Geometry: final body of the model. Coordinates: model frame, mm. Face numbers are marked on the shaded views. A direction names the side the tool comes from. Give positions to 0.01 mm unless a question says otherwise; leave off trailing zeros. Write each loop counter-clockwise with the first axis right and the second up, starting at its lowest first coordinate (ties: lowest second). Pieces come first, ordered by that corner, then holes.
Q1. Cut plane D-D on y = -16. Return the cut outline in (x, z).
Q2. Cut plane B-B on z = -2. Return the cut outline in (x, y).
Q3. Pin query (flat end, axial travel): pin 1 (11 mm diameter, centred on x = -47, y = 0, fed in from +Z); pin 2 (12 mm diameter, centred on x = 19.5, z = -46.5, fed in from +Y); pin 3 (14.5 mm diameter, centred on x = -48.5, y = -1, fed in from +Z); pin 4 (25 mm diameter, centred on x = 0, y = 0, fed in from +Z). Return the tip coordinate at first contact, or that it passes through.
Q4. Line query: L1, parallel to X at y = 0, z = -36; L2, parallel to Z at x = 24, y = 26.5; L3, parallel to Y at x = -47, z = -10.75. Output: solid intervals per line, ascending.
Q5. Cut plane C-C on z = -28.5. Return the cut outline in (x, y), plus the area to 3 significant figures.
Q6. Reachability of the marked faces 1, 2 and 3 from +Z, -Z, +X, -X, +Y, -Y: full face, straight path, thin tool, end or side. Return the list, or none.
Q7. Cut plane A-A on x = 0. Return the cut outline in (y, z), plus the area to 3 significant figures.
Q8. Draft query along X for the marked faces 4, 5 and 6. Return one class per face: pulls with the +X half, pulls with the -X half, needs draft (parallel to the pull), parting line crosses it, or undercut.
```python
from build123d import *

# Parameters (mm, degrees)
F0_R     = 27.5
F0_R_2   = 14
F1_DEPTH = 19
F2_DEPTH = 6
F3_R     = 27.5
F3_R_2   = 14
F4_DEPTH = 36
F5_R     = 5
F6_DEPTH = 25
F7_R     = 9
F8_DEPTH = 5


with BuildPart() as f1:
    # F0 (on Top) → F1 (new body)
    with BuildSketch(Plane.XY):
        with BuildLine():
            ThreePointArc((-33.8085106383, -9.0545352404), (-35, 0), (-33.8085106383, 9.0545352404))
            ThreePointArc((-33.8085106383, 9.0545352404), (-42.6314083028, 15.3920566067), (-53.4680851064, 14.6343389006))
            ThreePointArc((-53.4680851064, 14.6343389006), (-63, 0), (-53.4680851064, -14.6343389006))
            ThreePointArc((-53.4680851064, -14.6343389006), (-42.6314083028, -15.3920566067), (-33.8085106383, -9.0545352404))
        make_face()
        with BuildLine():
            ThreePointArc((-33.8085106383, 9.0545352404), (-26.5847239613, 22.7651587278), (-14.1489361702, 32.012616345))
            Line((-14.1489361702, 32.012616345), (-53.4680851064, 14.6343389006))
            ThreePointArc((-53.4680851064, 14.6343389006), (-42.6314083028, 15.3920566067), (-33.8085106383, 9.0545352404))
        make_face()
        with BuildLine():
            ThreePointArc((-31, 0), (-31.7182489585, 4.7400511713), (-33.8085106383, 9.0545352404))
            ThreePointArc((-33.8085106383, 9.0545352404), (-35, 0), (-33.8085106383, -9.0545352404))
            ThreePointArc((-33.8085106383, -9.0545352404), (-31.7182489585, -4.7400511713), (-31, 0))
        make_face()
        with BuildLine():
            ThreePointArc((33.8085106383, 9.0545352404), (26.5847239613, 22.7651587278), (14.1489361702, 32.012616345))
            ThreePointArc((14.1489361702, 32.012616345), (0, 35), (-14.1489361702, 32.012616345))
            ThreePointArc((-14.1489361702, 32.012616345), (-26.5847239613, 22.7651587278), (-33.8085106383, 9.0545352404))
            ThreePointArc((-33.8085106383, 9.0545352404), (-31.7182489585, 4.7400511713), (-31, 0))
            ThreePointArc((-31, 0), (-31.7182489585, -4.7400511713), (-33.8085106383, -9.0545352404))
            ThreePointArc((-33.8085106383, -9.0545352404), (-26.5847239613, -22.7651587278), (-14.1489361702, -32.012616345))
            ThreePointArc((-14.1489361702, -32.012616345), (0, -35), (14.1489361702, -32.012616345))
            ThreePointArc((14.1489361702, -32.012616345), (26.5847239613, -22.7651587278), (33.8085106383, -9.0545352404))
            ThreePointArc((33.8085106383, -9.0545352404), (31, 0), (33.8085106383, 9.0545352404))
        make_face()
        Circle(F0_R, mode=Mode.SUBTRACT)
        with BuildLine():
            ThreePointArc((-14.1489361702, -32.012616345), (-26.5847239613, -22.7651587278), (-33.8085106383, -9.0545352404))
            ThreePointArc((-33.8085106383, -9.0545352404), (-42.6314083028, -15.3920566067), (-53.4680851064, -14.6343389006))
            Line((-53.4680851064, -14.6343389006), (-14.1489361702, -32.012616345))
        make_face()
        Circle(F0_R)
        Circle(F0_R_2, mode=Mode.SUBTRACT)
        with BuildLine():
            ThreePointArc((53.4680851064, 14.6343389006), (42.6314083028, 15.3920566067), (33.8085106383, 9.0545352404))
            ThreePointArc((33.8085106383, 9.0545352404), (34.700849214, 4.5662965114), (35, 0))
            ThreePointArc((35, 0), (34.700849214, -4.5662965114), (33.8085106383, -9.0545352404))
            ThreePointArc((33.8085106383, -9.0545352404), (42.6314083028, -15.3920566067), (53.4680851064, -14.6343389006))
            ThreePointArc((53.4680851064, -14.6343389006), (60.4068893055, -8.7324291666), (63, 0))
            ThreePointArc((63, 0), (60.4068893055, 8.7324291666), (53.4680851064, 14.6343389006))
        make_face()
        with BuildLine():
            ThreePointArc((35, 0), (34.700849214, 4.5662965114), (33.8085106383, 9.0545352404))
            ThreePointArc((33.8085106383, 9.0545352404), (31, 0), (33.8085106383, -9.0545352404))
            ThreePointArc((33.8085106383, -9.0545352404), (34.700849214, -4.5662965114), (35, 0))
        make_face()
        with BuildLine():
            Line((53.4680851064, 14.6343389006), (14.1489361702, 32.012616345))
            ThreePointArc((14.1489361702, 32.012616345), (26.5847239613, 22.7651587278), (33.8085106383, 9.0545352404))
            ThreePointArc((33.8085106383, 9.0545352404), (42.6314083028, 15.3920566067), (53.4680851064, 14.6343389006))
        make_face()
        with BuildLine():
            ThreePointArc((53.4680851064, -14.6343389006), (42.6314083028, -15.3920566067), (33.8085106383, -9.0545352404))
            ThreePointArc((33.8085106383, -9.0545352404), (26.5847239613, -22.7651587278), (14.1489361702, -32.012616345))
            Line((14.1489361702, -32.012616345), (53.4680851064, -14.6343389006))
        make_face()
    extrude(amount=-F1_DEPTH)

    # F0 (on Top) → F2 (join)
    with BuildSketch(Plane.XY):
        Circle(F0_R)
        Circle(F0_R_2, mode=Mode.SUBTRACT)
    extrude(amount=F2_DEPTH)

    # F3 (on face) → F4 (join)
    with BuildSketch(Plane(origin=(0, 0, -19), x_dir=(1, 0, 0), z_dir=(0, 0, -1))):
        Circle(F3_R)
        Circle(F3_R_2, mode=Mode.SUBTRACT)
    extrude(amount=F4_DEPTH)

    # F5 (on face) → F6 (cut)
    with BuildSketch(Plane.XY):
        with Locations((-47, 0)):
            Circle(F5_R)
        with Locations((47, 0)):
            Circle(F5_R)
    extrude(amount=-F6_DEPTH, mode=Mode.SUBTRACT)

    # F7 (on face) → F8 (cut)
    with BuildSketch(Plane.XY):
        with Locations((-47, 0)):
            Circle(F7_R)
        with Locations((47, 0)):
            Circle(F7_R)
    extrude(amount=-F8_DEPTH, mode=Mode.SUBTRACT)


solid = f1.part
```
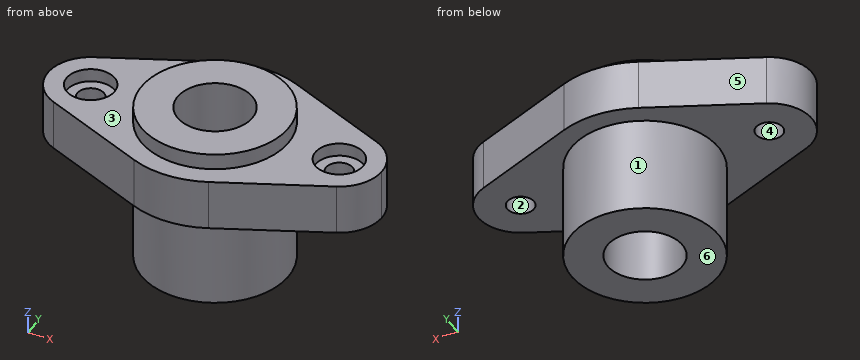
Data:
1. outline: (-50.38, -19) - (-22.37, -19) - (-22.37, -55) - (22.37, -55) - (22.37, -19) - (50.38, -19) - (50.38, 0) - (22.37, 0) - (22.37, 6) - (-22.37, 6) - (-22.37, 0) - (-50.38, 0) - close
2. outline: (-53.47, -14.63) - (-14.15, -32.01) arc R35 ccw to (14.15, -32.01) - (53.47, -14.63) arc R16 ccw to (53.47, 14.63) - (14.15, 32.01) arc R35 ccw to (-14.15, 32.01) - (-53.47, 14.63) arc R16 ccw to start; hole circle Ø18 at (-47, 0); hole circle Ø28 at (0, 0); hole circle Ø18 at (47, 0)
3. pin 1: stops at z = -5
3. pin 2: stops at y = 23.96
3. pin 3: stops at z = 0
3. pin 4: passes through
4. L1: x = -27.5 to -14, 14 to 27.5
4. L2: z = -19 to 0
4. L3: y = -17.49 to -5, 5 to 17.49
5. outline: circle Ø55 at (0, 0); hole circle Ø28 at (0, 0)
5. area: 1,760 mm2
6. face 1: -Z
6. face 2: +Z, -Z
6. face 3: +Z
7. outline: (-35, -19) - (-27.5, -19) - (-27.5, -55) - (-14, -55) - (-14, 6) - (-27.5, 6) - (-27.5, 0) - (-35, 0) - close; (14, -55) - (27.5, -55) - (27.5, -19) - (35, -19) - (35, 0) - (27.5, 0) - (27.5, 6) - (14, 6) - close
7. area: 1,930 mm2
8. face 4: undercut
8. face 5: pulls with the -X half
8. face 6: needs draft
